from build123d import *

# Parameters (mm, degrees)
BOSS_EXTRUDE1_DEPTH = 18
SKETCH2_R           = 1.75
CUT_EXTRUDE1_DEPTH  = 34
CUT_EXTRUDE2_DEPTH  = 1
CUT_EXTRUDE3_DEPTH  = 5


with BuildPart() as part:
    # Sketch1 → Boss-Extrude1 (new body)
    with BuildSketch(Plane(origin=(0, 0, 0), x_dir=(1, 0, 0), z_dir=(0, 1, 0))):
        with BuildLine():
            Line((-11.998275301, 32.528571429), (-29.498275301, 32.528571429))
            Line((-29.498275301, 32.528571429), (-29.498275301, 20.506241096))
            ThreePointArc((-29.498275301, 20.506241096), (-44.998275301, -7.471428571), (-29.498275301, -35.449098239))
            Line((-29.498275301, -35.449098239), (-29.498275301, -47.471428571))
            Line((-29.498275301, -47.471428571), (-11.998275301, -47.471428571))
            Line((-11.998275301, -47.471428571), (-11.998275301, -33.471428571))
            ThreePointArc((-11.998275301, -33.471428571), (-37.998275301, -7.471428571), (-11.998275301, 18.528571429))
            Line((-11.998275301, 18.528571429), (-11.998275301, 32.528571429))
        make_face()
    extrude(amount=BOSS_EXTRUDE1_DEPTH)

    # Sketch2 → Cut-Extrude1 (cut, through all)
    with BuildSketch(Plane(origin=(-11.998275301, 0, 0), x_dir=(0, 0, -1), z_dir=(1, 0, 0))):
        with Locations((-42.471428571, 5.25)):
            Circle(SKETCH2_R)
        with Locations((27.528571429, 5.25)):
            Circle(SKETCH2_R)
    extrude(amount=-CUT_EXTRUDE1_DEPTH, mode=Mode.SUBTRACT)

    # Sketch3 → Cut-Extrude2 (cut)
    with BuildSketch(Plane(origin=(-11.998275301, 0, 0), x_dir=(0, 0, -1), z_dir=(1, 0, 0))):
        Polygon((-45.326710591, 15.291960871), (-42.748719138, 15.291960871), (-42.748719138, 14.342174546), (-44.376924266, 14.342174546), (-44.376924266, 13.324546341), (-42.748719138, 13.324546341), (-42.748719138, 12.374760016), (-44.376924266, 12.374760016), (-44.376924266, 10.000294204), (-45.326710591, 10.000294204), align=None)
        Polygon((-41.231817095, 15.291960871), (-39.763676403, 15.291960871), (-39.763676403, 10.000294204), (-40.713462728, 10.000294204), (-40.713462728, 14.410016426), (-41.798932813, 14.410016426), align=None)
        with BuildLine():
            add(Edge.make_bspline(
                [(-36.353561886, 15.427644632), (-36.307588286, 15.42696214), (-36.217191905, 15.425620181), (-36.084055051, 15.411085663), (-35.955807451, 15.389128061), (-35.831947383, 15.358504863), (-35.713366407, 15.317976152), (-35.599201463, 15.269463978), (-35.490811447, 15.21042378), (-35.386814038, 15.143734844), (-35.287249296, 15.068233514), (-35.194510191, 14.9821581), (-35.106903109, 14.8874892), (-35.026324422, 14.78279559), (-34.950989689, 14.66902957), (-34.881146448, 14.546173101), (-34.817329365, 14.413624881), (-34.758823205, 14.271145717), (-34.706506811, 14.116599909), (-34.662440778, 13.948214748), (-34.624646781, 13.765951781), (-34.592745981, 13.569357327), (-34.568634132, 13.358170067), (-34.55238226, 13.132530302), (-34.541229457, 12.892873032), (-34.540319242, 12.728470114), (-34.539851616, 12.644007479)],
                knots=[0, 0, 0, 0, 0.000137869, 0.000271087, 0.000401268, 0.000528016, 0.000653387, 0.000776847, 0.000899687, 0.001023184, 0.001147212, 0.001273995, 0.001402276, 0.001533737, 0.001669859, 0.001811332, 0.001957355, 0.002110898, 0.002273142, 0.002446443, 0.002632718, 0.002831386, 0.003043736, 0.003270158, 0.003509959, 0.003763326, 0.003763326, 0.003763326, 0.003763326], degree=3))
            add(Edge.make_bspline(
                [(-34.539851616, 12.644007479), (-34.540356994, 12.558488121), (-34.541338933, 12.392325544), (-34.551918635, 12.150476247), (-34.570137381, 11.923198201), (-34.593619017, 11.710514921), (-34.625782434, 11.51253872), (-34.663450266, 11.328756974), (-34.708211869, 11.159236299), (-34.762251547, 11.004358661), (-34.820403569, 10.861629272), (-34.884395218, 10.72933949), (-34.95311113, 10.607131), (-35.024975169, 10.49316012), (-35.103927185, 10.390786655), (-35.186124362, 10.296529371), (-35.275145712, 10.213978649), (-35.36724309, 10.138880195), (-35.465790398, 10.07398006), (-35.569771342, 10.017219472), (-35.681039722, 9.971179894), (-35.797567305, 9.931137128), (-35.921340327, 9.902390743), (-36.050392052, 9.87958143), (-36.186179447, 9.866975605), (-36.278628975, 9.86541177), (-36.326001122, 9.864610443)],
                knots=[0, 0, 0, 0, 0.000256547, 0.000498466, 0.000726027, 0.000940483, 0.001140197, 0.00132751, 0.001503133, 0.001665719, 0.001819262, 0.001965285, 0.002106237, 0.002239733, 0.002369061, 0.002493713, 0.002614449, 0.002732817, 0.002849829, 0.002967931, 0.003087634, 0.003210657, 0.003337152, 0.003468377, 0.003603601, 0.003745708, 0.003745708, 0.003745708, 0.003745708], degree=3))
            add(Edge.make_bspline(
                [(-36.326001122, 9.864610443), (-36.373371991, 9.865427227), (-36.466170825, 9.867027294), (-36.602325403, 9.879487701), (-36.732061037, 9.902483144), (-36.856813303, 9.931357822), (-36.975713944, 9.971091296), (-37.089333085, 10.018508345), (-37.196797094, 10.074914775), (-37.298403521, 10.139966121), (-37.393805453, 10.214562109), (-37.484485436, 10.297904852), (-37.57024288, 10.389783097), (-37.649773202, 10.491225956), (-37.724378878, 10.600879379), (-37.793281889, 10.719995555), (-37.856440827, 10.848401053), (-37.915831314, 10.986274857), (-37.96743413, 11.136585233), (-38.01335824, 11.300674432), (-38.050978063, 11.479910274), (-38.081234442, 11.674235178), (-38.105391117, 11.883237456), (-38.123360907, 12.10701799), (-38.133999374, 12.34568101), (-38.134971016, 12.509725991), (-38.135471275, 12.594186098)],
                knots=[0, 0, 0, 0, 0.000142107, 0.000278386, 0.000409611, 0.000537137, 0.000662171, 0.000785217, 0.000906125, 0.0010258, 0.001146662, 0.001268952, 0.001394958, 0.001523261, 0.001655272, 0.00179254, 0.001935707, 0.002084361, 0.002242593, 0.002412082, 0.002595246, 0.002791652, 0.003001896, 0.003226287, 0.003465029, 0.003718396, 0.003718396, 0.003718396, 0.003718396], degree=3))
            add(Edge.make_bspline(
                [(-38.135471275, 12.594186098), (-38.134565103, 12.711536767), (-38.132816632, 12.937966394), (-38.11065873, 13.265091372), (-38.078136549, 13.567461747), (-38.03036917, 13.844571729), (-37.971305466, 14.097447652), (-37.895671318, 14.324423703), (-37.809567342, 14.528640603), (-37.736195692, 14.649619924), (-37.700859229, 14.707884682)],
                knots=[0, 0, 0, 0, 0.000351987, 0.000679164, 0.000983171, 0.00126392, 0.001522311, 0.001761317, 0.001981101, 0.002185291, 0.002185291, 0.002185291, 0.002185291], degree=3))
            add(Edge.make_bspline(
                [(-37.700859229, 14.707884682), (-37.659771672, 14.765123962), (-37.579437402, 14.877038034), (-37.438970685, 15.023960291), (-37.288057486, 15.149615399), (-37.123598134, 15.251159672), (-36.948193623, 15.331237493), (-36.760338015, 15.387795557), (-36.560725029, 15.42074892), (-36.423647462, 15.425311736), (-36.353561886, 15.427644632)],
                knots=[0, 0, 0, 0, 0.000211159, 0.000412857, 0.000607894, 0.000798799, 0.000990925, 0.001184751, 0.001385682, 0.001595891, 0.001595891, 0.001595891, 0.001595891], degree=3))
        make_face()
        with BuildLine():
            add(Edge.make_bspline(
                [(-36.33024124, 14.477858307), (-36.371801756, 14.475888421), (-36.453282428, 14.472026399), (-36.571514767, 14.439243282), (-36.68300048, 14.38860799), (-36.767804684, 14.327676333), (-36.831279787, 14.269266033), (-36.875630297, 14.216406611), (-36.918399374, 14.157419305), (-36.956175176, 14.089642323), (-36.991845394, 14.01551097), (-37.026705949, 13.934688735), (-37.055282451, 13.84519045), (-37.083358105, 13.74854028), (-37.107954999, 13.642066107), (-37.128561803, 13.524897621), (-37.146972171, 13.396272864), (-37.159813623, 13.256107588), (-37.171785709, 13.10454844), (-37.180367868, 12.941257804), (-37.183955853, 12.766279733), (-37.185096364, 12.645774932), (-37.18568495, 12.583585804)],
                knots=[0, 0, 0, 0, 0.000124476, 0.000244038, 0.000365457, 0.000490162, 0.000555412, 0.000623823, 0.000696773, 0.000773689, 0.000856181, 0.000943593, 0.001037452, 0.001137775, 0.001245513, 0.001365071, 0.001494594, 0.001635195, 0.001787227, 0.001950691, 0.002125648, 0.002312225, 0.002312225, 0.002312225, 0.002312225], degree=3))
            add(Edge.make_bspline(
                [(-37.18568495, 12.583585804), (-37.184716209, 12.503016782), (-37.182858577, 12.348519708), (-37.173129169, 12.126347537), (-37.153627378, 11.924152971), (-37.129371087, 11.740565663), (-37.095302136, 11.576776226), (-37.056103602, 11.43123506), (-37.007696898, 11.305797462), (-36.951753625, 11.198649322), (-36.88979393, 11.107498621), (-36.822533954, 11.030020115), (-36.752263661, 10.962927384), (-36.676789684, 10.908428786), (-36.596292083, 10.866663572), (-36.511442865, 10.83662237), (-36.422188108, 10.818232899), (-36.361067371, 10.81568287), (-36.33024124, 10.814396768)],
                knots=[0, 0, 0, 0, 0.000241724, 0.000463523, 0.000666886, 0.000850978, 0.001018747, 0.001168433, 0.001302685, 0.001421223, 0.001530303, 0.001632518, 0.001728508, 0.001821174, 0.001910782, 0.001999629, 0.002090477, 0.002182918, 0.002182918, 0.002182918, 0.002182918], degree=3))
            add(Edge.make_bspline(
                [(-36.33024124, 10.814396768), (-36.300472964, 10.815276815), (-36.242190381, 10.816999837), (-36.157201323, 10.834686425), (-36.07682963, 10.863440976), (-36.00131797, 10.904116306), (-35.930396249, 10.955841213), (-35.864411087, 11.018842997), (-35.803860132, 11.093749638), (-35.768582871, 11.149341444), (-35.750405169, 11.177986846)],
                knots=[0, 0, 0, 0, 8.92e-05, 0.000174643, 0.00025914, 0.000344503, 0.000431011, 0.000521735, 0.000617426, 0.00071915, 0.00071915, 0.00071915, 0.00071915], degree=3))
            add(Edge.make_bspline(
                [(-35.750405169, 11.177986846), (-35.729003986, 11.217129871), (-35.684127441, 11.299209621), (-35.632196225, 11.437716138), (-35.588483423, 11.593928598), (-35.550860453, 11.768333148), (-35.525128636, 11.961617661), (-35.502968427, 12.172556504), (-35.492280008, 12.402211879), (-35.490541478, 12.561317951), (-35.489637941, 12.644007479)],
                knots=[0, 0, 0, 0, 0.000133698, 0.000280354, 0.000442414, 0.000620174, 0.000815058, 0.001027066, 0.001256329, 0.001504413, 0.001504413, 0.001504413, 0.001504413], degree=3))
            add(Edge.make_bspline(
                [(-35.489637941, 12.644007479), (-35.489986958, 12.727414792), (-35.490658756, 12.88795963), (-35.502984298, 13.118440632), (-35.520148556, 13.328946776), (-35.545254912, 13.519008087), (-35.577558802, 13.68908595), (-35.617373468, 13.839169248), (-35.664311998, 13.969553765), (-35.719975501, 14.080109491), (-35.781626288, 14.174066693), (-35.847070481, 14.254674684), (-35.916584804, 14.323495752), (-35.990053007, 14.380788885), (-36.069175537, 14.424565135), (-36.152441049, 14.45547479), (-36.240020246, 14.474174094), (-36.299761657, 14.47661366), (-36.33024124, 14.477858307)],
                knots=[0, 0, 0, 0, 0.000250187, 0.000481568, 0.000692226, 0.000883669, 0.001056428, 0.001211224, 0.001349065, 0.001471373, 0.001581627, 0.001685596, 0.001782291, 0.00187452, 0.001964197, 0.002052409, 0.002140142, 0.002231527, 0.002231527, 0.002231527, 0.002231527], degree=3))
        make_face(mode=Mode.SUBTRACT)
    extrude(amount=-CUT_EXTRUDE2_DEPTH, mode=Mode.SUBTRACT)

    # Sketch4 → Cut-Extrude3 (cut)
    with BuildSketch(Plane.ZY.offset(29.498275301)):
        Polygon((-25.391799088, 2.901056132), (-24.425940196, 5.926027195), (-26.562712537, 8.274971063), (-29.665343769, 7.598943868), (-30.631202661, 4.573972805), (-28.49443032, 2.225028937), align=None)
        Polygon((44.716794169, 3.004634402), (45.538655018, 6.071860849), (43.293289421, 8.317226447), (40.226062974, 7.495365598), (39.404202124, 4.428139151), (41.649567722, 2.182773553), align=None)
    extrude(amount=-CUT_EXTRUDE3_DEPTH, mode=Mode.SUBTRACT)


solid = part.part
Work out the finished part from the listing and answer in its coordinate system (mm). A direction names the side the tool comes from. Coordinates: 2 decimals unless noted, no trailing zeros. Write each loop counter-clockwise with the first axis right and the second up, starting at its lowest first coordinate (ties: lowest second). Pieces come first, ordered by that corner, then holes. Notation, with made-up numbers: M -35,47.5 L -13,47.5 A23 ccw -13,76.5 Z; hole C -35.75,74.25 d3. An arc over 180 degrees is marked long. Write item = value, one per line.
1. For faces 1 (the face through (-27.033, 4.392, -24.916)), 2 (the face through (-12.998, 13, 35)), 3 (the face through (-29.498, 9, -27)), 4 (the face through (-44.995, 8.874, 7.004)), determine the directions among +Z, -Z, +X, -X, +Y, -Y from which every point of the face is accessible in a straight line to the end or side of a thin tool.
Solution:
face_1 = -X
face_2 = +X
face_3 = -Z, -X, +Y, -Y
face_4 = -X, +Y, -Y
2. Determine the mould class of faces 5 (the face through (-18.16, 5.33, 44.22)), 6 (the face through (-40, 0, 7)), 7 (the face through (-11.998, 9, -25)) for opening direction Y: released by +Y, released by -Y, zero draft, split by the parting line, or undercut.
Solution:
face_5 = undercut
face_6 = released by -Y
face_7 = zero draft
3. Straight lines are drawn through the part: line 1 (Z direction, x = -28.5, y = 4); line 2 (Z direction, x = -28.5, y = 6); line 3 (Z direction, x = -31.5, y = 1.5). For each, find the intervals that lie inside material, in ascending order. Write a range as from..to.
Solution:
line_1 = -32.53..-30.11, -25.04..-12.62, 27.56..39.83, 44.98..47.47
line_2 = -32.53..-30.18, -24.49..-12.62, 27.56..39.83, 45.52..47.47
line_3 = -19.15..-9.72, 24.67..34.09
4. The part is cut by section B-B (x = -35.5). Determine the outline of the cut face in (y, z), then the cut area to 3 significant figures.
Solution:
outline = M 0,-15.69 L 18,-15.69 L 18,-3.65 L 0,-3.65 Z; M 0,18.59 L 18,18.59 L 18,30.64 L 0,30.64 Z
area = 434 mm2
5. The part is cut by section C-C (x = -20). Determine the outline of the cut face in (y, z).
Solution:
outline = M 0,-32.53 L 18,-32.53 L 18,-17.27 L 0,-17.27 Z; M 0,32.21 L 18,32.21 L 18,47.47 L 0,47.47 Z; hole C 5.25,-27.53 d3.5; hole C 5.25,42.47 d3.5
6. The part is cut by section A-A (x = -15). Determine the outline of the cut face in (y, z).
Solution:
outline = M 0,-32.53 L 18,-32.53 L 18,-18.35 L 0,-18.35 Z; M 0,33.3 L 18,33.3 L 18,47.47 L 0,47.47 Z; hole C 5.25,-27.53 d3.5; hole C 5.25,42.47 d3.5
7. The part is cut by section D-D (x = -30.5). Determine the outline of the cut face in (y, z), then the cut area to 3 significant figures.
Solution:
outline = M 0,-19.85 L 18,-19.85 L 18,-10.8 L 0,-10.8 Z; M 0,25.74 L 18,25.74 L 18,34.8 L 0,34.8 Z
area = 326 mm2
8. Flat-ended cylindrical pins translate along their axes: pin 1 (2 mm diameter, centred on y = 5.25, z = 42.47, fed in from +X); pin 2 (5 mm diameter, centred on y = 8, z = 12.5, fed in from -X); pin 3 (6.5 mm diameter, centred on y = 6, z = 43, fed in from -X); pin 4 (4 mm diameter, centred on y = 4, z = 7.5, fed in from +X). Find the tip coordinate at first contact, or state that the pin passes through.
Solution:
pin_1 = through
pin_2 = -44.9
pin_3 = -29.5
pin_4 = -37.92
